```python
from build123d import *

# Parameters (mm, degrees)
BOSS_EXTRUDE1_START     = 50
BOSS_EXTRUDE1_DEPTH     = 3
BOSS_EXTRUDE2_DEPTH     = 3
CUT_EXTRUDE1_DEPTH      = 145.867832485
CUT_EXTRUDE1_DEPTH_BACK = 145.867832485
SKETCH2_R               = 1.5
SKETCH3_W               = 56
SKETCH3_H               = 20
BOSS_EXTRUDE4_DEPTH     = 3
SKETCH4_W               = 56
SKETCH4_H               = 20
BOSS_EXTRUDE5_DEPTH     = 3


with BuildPart() as part:
    # Sketch1 → Boss-Extrude1 (new body)
    with BuildSketch(Plane.XY.offset(BOSS_EXTRUDE1_START)):
        with BuildLine():
            Line((-10, 133.333), (10, 133.333))
            ThreePointArc((10, 133.333), (17.071067812, 130.404067812), (20, 123.333))
            Line((20, 123.333), (20, -123.333))
            ThreePointArc((20, -123.333), (17.071067812, -130.404067812), (10, -133.333))
            Line((10, -133.333), (-10, -133.333))
            ThreePointArc((-10, -133.333), (-17.071067812, -130.404067812), (-20, -123.333))
            Line((-20, -123.333), (-20, 123.333))
            ThreePointArc((-20, 123.333), (-17.071067812, 130.404067812), (-10, 133.333))
        make_face()
    extrude(amount=BOSS_EXTRUDE1_DEPTH)


with BuildPart() as body_2:
    # Sketch1_3 → Boss-Extrude2 (new body)
    with BuildSketch(Plane.XY):
        with BuildLine():
            Line((-10, 133.333), (10, 133.333))
            ThreePointArc((10, 133.333), (17.071067812, 130.404067812), (20, 123.333))
            Line((20, 123.333), (20, -123.333))
            ThreePointArc((20, -123.333), (17.071067812, -130.404067812), (10, -133.333))
            Line((10, -133.333), (-10, -133.333))
            ThreePointArc((-10, -133.333), (-17.071067812, -130.404067812), (-20, -123.333))
            Line((-20, -123.333), (-20, 123.333))
            ThreePointArc((-20, 123.333), (-17.071067812, 130.404067812), (-10, 133.333))
        make_face()
    extrude(amount=-BOSS_EXTRUDE2_DEPTH)


with BuildPart() as cut_extrude1_tool:
    # Sketch2 → Cut-Extrude1 (new, two sides: drawn at the far end of the back side and taken through both)
    with BuildSketch(Plane.XY.offset(-CUT_EXTRUDE1_DEPTH_BACK)):
        with Locations((0, 119.997946932)):
            Circle(SKETCH2_R)
        with Locations(Location((0, -119.997946932, 0), (0, 0, 180))):
            Circle(SKETCH2_R)
    extrude(amount=CUT_EXTRUDE1_DEPTH + CUT_EXTRUDE1_DEPTH_BACK)


with BuildPart() as part_1:
    add(part.part)

    # Cut-Extrude1: cut by cut_extrude1_tool
    add(cut_extrude1_tool.part, mode=Mode.SUBTRACT)



with BuildPart() as body_2_1:
    add(body_2.part)

    # Cut-Extrude1: cut by cut_extrude1_tool
    add(cut_extrude1_tool.part, mode=Mode.SUBTRACT)


with BuildPart() as part_2:
    add(part_1.part)

    add(body_2_1.part)  # Boss-Extrude4 merges body 2
    # Sketch3 → Boss-Extrude4 (add)
    with BuildSketch(Plane.ZY.offset(20)):
        with Locations((25, 108.333)):
            Rectangle(SKETCH3_W, SKETCH3_H)
        with Locations((25, 68.333)):
            Rectangle(SKETCH3_W, SKETCH3_H)
        with Locations((25, 28.333)):
            Rectangle(SKETCH3_W, SKETCH3_H)
        with Locations((25, -11.667)):
            Rectangle(SKETCH3_W, SKETCH3_H)
        with Locations((25, -51.667)):
            Rectangle(SKETCH3_W, SKETCH3_H)
        with Locations((25, -91.667)):
            Rectangle(SKETCH3_W, SKETCH3_H)
    extrude(amount=BOSS_EXTRUDE4_DEPTH)

    # Sketch4 → Boss-Extrude5 (add)
    with BuildSketch(Plane(origin=(20, 0, 0), x_dir=(0, 0, -1), z_dir=(1, 0, 0))):
        with Locations((-25, -51.667)):
            Rectangle(SKETCH4_W, SKETCH4_H)
        with Locations((-25, -11.667)):
            Rectangle(SKETCH4_W, SKETCH4_H)
        with Locations((-25, -91.667)):
            Rectangle(SKETCH4_W, SKETCH4_H)
    extrude(amount=BOSS_EXTRUDE5_DEPTH)


solid = part_2.part
```
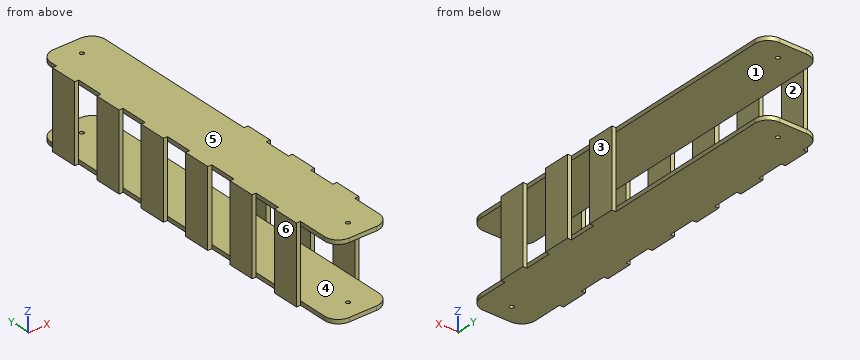
Work out the finished part from the listing and answer in its coordinate system (mm). Face numbers are marked on the shaded views. A direction names the side the tool comes from. Give positions to 0.01 mm unless a question says otherwise; leave off trailing zeros. Loops run counter-clockwise (first coordinate to the right, second up) from the corner with the lowest first, then second, coordinate; pieces in that order, holes last. Notation, with made-up numbers: (73, -29) -> (109, -29) arc R23 cw to (109, -8) -> close; hole circle Ø9 at (31.5, -39.75). An arc over 180 degrees is marked (long way). One line per question, with ' | ' between items. Start each with the question number.
1) Section C-C, the plane z = 34 is taken. State how many separate pieces and enclosed holes the cut face has, then the cut area to 3 significant figures.
2) Section B-B, the plane x = 17 is taken. Determine the outline of the cut face in (y, z).
3) Each of these flat-tipped pins is pushed along its axis until it touches: pin 1 (2.5 mm diameter, centred on y = -115, z = -2, fed in from -X); pin 2 (3.5 mm diameter, centred on x = -22, z = 22.5, fed in from +Y); pin 3 (3.5 mm diameter, centred on x = 21.5, z = 35.5, fed in from -Y). Where does it stop, or does it pass through?
4) Section D-D, the plane y = 111 is taken. Determine the outline of the cut face in (x, z), then the cut area to 3 significant figures.
5) Determine the mould class of the marked faces 4, 5 and 6 for opening direction X: +X half, -X half, draft (parallel to the pull), parting line (faces both ways), or undercut.
6) For the marked faces 1, 2 and 3, determine the directions among +Z, -Z, +X, -X, +Y, -Y from which every point of the face is accessible in a straight line to the end or side of a thin tool.
7) Section A-A, the plane y = -25 is taken. Determine the outline of the cut face in (x, z).
8) Straight lines are drawn through the part: L1, parallel to Y at x = 0, z = -1; L2, parallel to X at y = -83.5, z = 48.5; L3, parallel to Z at x = 0, y = 100. For each, find the intervals that lie inside material, in ascending order.
Resolved:
1) separate pieces: 9 | enclosed holes: 0 | area: 540 mm2
2) outline: (-130.47, -3) -> (130.47, -3) -> (130.47, 0) -> (-130.47, 0) -> close; (-130.47, 50) -> (130.47, 50) -> (130.47, 53) -> (-130.47, 53) -> close
3) pin 1: x = -20 | pin 2: y = 118.33 | pin 3: y = -101.67
4) outline: (-23, -3) -> (20, -3) -> (20, 0) -> (-20, 0) -> (-20, 50) -> (20, 50) -> (20, 53) -> (-23, 53) -> close | area: 408 mm2
5) face 4: undercut | face 5: draft | face 6: -X half
6) face 1: +Y, -Y | face 2: +X, +Y, -Y | face 3: +Z, -Z, +X, +Y, -Y
7) outline: (-20, -3) -> (20, -3) -> (20, 0) -> (-20, 0) -> close; (-20, 50) -> (20, 50) -> (20, 53) -> (-20, 53) -> close
8) L1: -133.33 to -121.5, -118.5 to 118.5, 121.5 to 133.33 | L2: -23 to -20, 20 to 23 | L3: -3 to 0, 50 to 53
